Verification items for the finished model (mm, model axes). Round coordinates to 2 decimals unless told otherwise and drop trailing zeros. Loops run counter-clockwise (first coordinate to the right, second up) from the corner with the lowest first, then second, coordinate; pieces in that order, holes last. Notation, with made-up numbers: M 10.25,64.5 L 19.25,64.5 A4 ccw 19.25,70.5 Z; hole C 74,76 d8. An arc over 180 degrees is marked long. Write item = value, one per line. Start each with the question number.
from build123d import *


with BuildPart() as part:
    # Sketch2 → Revolve1 (revolve)
    with BuildSketch(Plane(origin=(0, 0, 0), x_dir=(0, 0, -1), z_dir=(1, 0, 0))):
        with BuildLine():
            Line((-0.34, 3), (-0.34, 5.4))
            Line((-0.34, 5.4), (-0.44, 5.4))
            ThreePointArc((-0.44, 5.4), (-0.67, 5.249201276), (-0.9, 5.4))
            Line((-0.9, 5.4), (-1, 5.4))
            Line((-1, 5.4), (-1, 3))
            Line((-1, 3), (-0.34, 3))
        make_face()
    revolve1 = revolve(axis=Axis((0, 0, 3.014677367), (0, 0, -1)))

    # Mirror2: Revolve1 across plane
    add(revolve1.mirror(Plane(origin=(0, 0, 0.34), x_dir=(1, 0, 0), z_dir=(0, 0, -1))))

    # Mirror3: Revolve1 across plane
    add(revolve1.mirror(Plane.XY.offset(1)))


solid = part.part
1. Section check A-A, the plane y = 0. Enter the section's corners in (x, z).
2. Thickness scan on line 1 (X direction, y = -2.25, z = 0.4); line 2 (X direction, y = 0, z = 0.15); line 3 (Y direction, x = -2.25, z = 0.75). Record the ranges inside material, lowest first.
Computed values:
q1.outline = M -5.4,-0.32 L -3,-0.32 L -3,1.66 L -5.4,1.66 L -5.4,1.56 A0.25 cw -5.4,1.1 L -5.4,0.9 A0.25 cw -5.4,0.44 L -5.4,0.24 A0.25 cw -5.4,-0.22 Z; M 3,-0.32 L 5.4,-0.32 L 5.4,-0.22 A0.25 cw 5.4,0.24 L 5.4,0.44 A0.25 cw 5.4,0.9 L 5.4,1.1 A0.25 cw 5.4,1.56 L 5.4,1.66 L 3,1.66 Z
q2.line_1 = -4.91 to -1.98, 1.98 to 4.91
q2.line_2 = -5.29 to -3, 3 to 5.29
q2.line_3 = -4.76 to -1.98, 1.98 to 4.76
